Autodesk Inventor part; units mm, degrees
ref_plane "YZ Plane" through (0, 0, 0) normal (1, 0, 0) x (0, 1, 0)
ref_plane "XZ Plane" through (0, 0, 0) normal (0, 1, 0) x (-1, 0, 0)
ref_plane "XY Plane" through (0, 0, 0) normal (0, 0, 1) x (1, 0, 0)
sketch "Sketch1" plane through (0, 0, 0) normal (1, 0, 0) x (0, 1, 0)
  line L0 (0, 0) -> (15, -5.4596)
  line L1 (0, 0) -> (0, -9.4596)
  line L2 (15, -5.4596) -> (15, -9.4596)
  line L3 (15, -9.4596) -> (0, -9.4596)
  dimension "d12" = 70
  dimension "d17" = 15
  dimension "d18" = 4
extrude "Extrusion1" add sketch "Sketch1" along normal blind 7.5
sketch "Sketch2" plane through (7.5, 0, 0) normal (1, 0, 0) x (0, 0, -1)
  line L0 (9.4596, 0) -> (9.4596, 15)
  line L1 (9.4596, 1) -> (1.4596, 1)
  line L2 (0, 0) -> (9.4596, 0)
  line L3 (1.4596, 1) -> (4.7353, 10)
  line L4 (9.4596, 10) -> (4.7353, 10)
  line L5 (9.4596, 1) -> (9.4596, 10)
  point P0 (5.4596, 15)
  dimension "d23" = 8
  dimension "d24" = 10
  dimension "d25" = 70
  dimension "d26" = 4.7243
extrude "Extrusion2" cut sketch "Sketch2" against normal blind 10
sketch "Sketch5" plane through (0, 0, 0) normal (-1, 0, 0) x (0, 0, 1)
  line L0 (-5.4596, 15) -> (-9.4596, 15)
  line L1 (-9.4596, 10) -> (-4.7353, 10)
  line L2 (-4.7353, 10) -> (-1.4596, 1)
  line L3 (-1.4596, 1) -> (-9.4596, 1)
  line L4 (-9.4596, 1) -> (-9.4596, 0)
  line L5 (-9.4596, 0) -> (0, 0)
  line L6 (0, 0) -> (-5.4596, 15)
  line L7 (-5.4596, 15) -> (-9.4596, 15)
  line L8 (-9.4596, 15) -> (-9.4596, 10)
  line L9 (-9.4596, 10) -> (-11.2794, 15)
  line L10 (-5.4596, 15) -> (0, 0)
  line L11 (-9.4596, 10) -> (-9.4596, 15)
  line L12 (-9.4596, 10) -> (-9.4596, 15)
  line L13 (-9.4596, 15) -> (-11.2794, 15)
extrude "Extrusion5" add sketch "Sketch5" against normal up to surface (7.5 mm away) contours L8 L9 L13
sketch "Sketch6" plane through (7.5, 0, 0) normal (1, 0, 0) x (0, 0, -1)
  line L0 (5.4596, 15) -> (0, 0)
  line L1 (0, 0) -> (-0.364, -1)
  line L2 (9.4596, 0) -> (9.4596, 1)
  line L3 (9.4596, 0) -> (9.4596, -1)
  line L4 (0, 0) -> (9.4596, 0)
  line L5 (0, 0) -> (9.4596, 0)
  line L6 (9.4596, -1) -> (-0.364, -1)
  dimension "d41" = 1
  dimension "d42" = 70
extrude "Extrusion6" add sketch "Sketch6" against normal up to surface (7.5 mm away)
sketch "Sketch4" plane through (7.5, 1, -1.4596) normal (0, 1, 0) x (1, 0, 0)
  line L0 (-7.5, 0) -> (-7.5, 8)
  line L1 (-7.5, 8) -> (0, 8)
  circle A0 centre (-3.75, 4) radius 1.75
  point P0 (-7.5, -1.4596)
  point P1 (-7.5, 4)
  point P2 (-3.75, 8)
  dimension "d32" = 3.5
extrude "Extrusion4" cut sketch "Sketch4" against normal blind 10
sketch "Sketch7" plane through (7.5, 0, 0) normal (1, 0, 0) x (0, 0, -1)
  line L0 (5.4596, 15) -> (11.2794, 15)
  line L1 (-0.364, -1) -> (9.4596, -1)
  line L2 (5.4596, 15) -> (4.4596, 15)
  line L3 (-0.364, -1) -> (-1.364, -1)
  line L4 (-1.364, -1) -> (4.4596, 15)
  line L5 (5.4596, 15) -> (-0.364, -1)
  line L6 (5.4596, 15) -> (-0.364, -1)
  point P0 (0, 0)
  dimension "d45" = 1
  dimension "d46" = 1
extrude "Extrusion7" add sketch "Sketch7" against normal up to surface (7.5 mm away)
sketch "Sketch3" plane through (7.5, 15, -9.4596) normal (0, 0, -1) x (-1, 0, 0)
  circle A0 centre (3.75, -2.5) radius 1.75
  line L0 (7.5, 0) -> (0, 0)
  line L1 (7.5, 0) -> (7.5, -5)
  point P0 (7.5, -15)
  point P1 (3.75, 0)
  point P2 (7.5, -2.5)
  dimension "d29" = 3.5
extrude "Extrusion3" cut sketch "Sketch3" against normal blind 10 and the other way blind 5
properties part number "camera-brackets-angle"
For this review, take the finished solid that the model builds, in its own axes (mm). A direction names the side the tool comes from. Coordinates: 2 decimals unless noted, no trailing zeros. Loops run counter-clockwise (first coordinate to the right, second up) from the corner with the lowest first, then second, coordinate; pieces in that order, holes last. Notation, with made-up numbers: (12, -9) -> (56, -9) arc R4 cw to (56, -2) -> close; hole circle Ø3 at (38.5, -31.75). An arc over 180 degrees is marked (long way). Return JSON: item names as keys, results as strings. Group by question number.
(1) Consider section D-D, the plane x = 3.75. Give the boundary of the cut face in (y, z), plus the area to 3 significant figures.
(2) For pin 1 Ø0.6 at (x, y) = (4.5, -0.5) entering from -Z; pin 2 Ø4.5 at (x, y) = (3.75, 12.5) entering from -Z; pin 3 Ø1 at (x, y) = (3, 7) entering from -Z, all flat-tipped, find the tip position at first contact; note any pin that passes through.
(3) Consider section A-A, the plane z = -1.75. Give the boundary of the cut face in (x, y), plus the area to 3 significant figures.
(4) Consider section C-C, the plane y = 12.5. Give the boundary of the cut face in (x, z), plus the area to 3 significant figures.
(5) Mouldability with a two-part tool opening along Y and no side actions: class faces 1 (the flat face through (4, 15, -8)), 2 (the flat face through (0, 9, -4)), 3 (the cylindrical face through (4.13, 10.79, -7.02)) as pulls with the +Y half, pulls with the -Y half, needs draft (parallel to the pull), parting line crosses it, or undercut.
(6) Consider section B-B, the plane x = 1. Give the boundary of the cut face in (y, z).
(7) To check wall thickness, follow L1, parallel to Y at x = 3.75, z = -8.75; L2, parallel to Y at x = 1.75, z = -9; L3, parallel to X at y = 12.5, z = -9. State the ranges of each line that lie inside material, in increasing order.
(8) Tool access review of faces 4 (the flat face through (3.802, 5.437, -3.075)), 5 (the cylindrical face through (2.46, 0.01, -6.64)), 6 (the flat face through (4, 0, -9.46)): name each direction out of +Z, -Z, +X, -X, +Y, -Y from which nothing blocks a thin tool from reaching the whole face with its end or side.
Results below:
{
 "1": {"outline": "(-1, -9.46) -> (1, -9.46) -> (1, -7.21) -> (-1, -7.21) -> close; (-1, -3.71) -> (1, -3.71) -> (1, -1.46) -> (10, -4.74) -> (10, -9.46) -> (10.75, -9.73) -> (10.75, -2.91) -> (-1, 1.36) -> close; (14.25, -11.01) -> (15, -11.28) -> (15, -4.46) -> (14.25, -4.19) -> close", "area": "43.0 mm2"},
 "2": {"pin 1": "stops at z = -9.46", "pin 2": "stops at z = -11.19", "pin 3": "stops at z = -3.83"},
 "3": {"outline": "(0, -1) -> (7.5, -1) -> (7.5, 1) -> (0, 1) -> close; (0, 1.8) -> (7.5, 1.8) -> (7.5, 7.56) -> (0, 7.56) -> close", "area": "58.2 mm2"},
 "4": {"outline": "(0, -10.37) -> (2, -10.37) -> (2, -3.55) -> (0, -3.55) -> close; (5.5, -10.37) -> (7.5, -10.37) -> (7.5, -3.55) -> (5.5, -3.55) -> close", "area": "27.3 mm2"},
 "5": {"face 1": "pulls with the +Y half", "face 2": "needs draft", "face 3": "undercut"},
 "6": {"outline": "(-1, -9.46) -> (1, -9.46) -> (1, -1.46) -> (10, -4.74) -> (10, -9.46) -> (15, -11.28) -> (15, -4.46) -> (-1, 1.36) -> close"},
 "7": {"L1": "y = -1 to 1, 10 to 10.75, 14.25 to 15", "L2": "y = -1 to 1, 10 to 15", "L3": "x = 0 to 2, 5.5 to 7.5"},
 "8": {"face 4": "-Z, +X, -X", "face 5": "-Y", "face 6": "-Z, +X, -X, -Y"}
}
